Geometry: see drawing. Coordinates: mm, zero at the bounding-box minimum. A direction names the side the tool comes from. Coordinates: 2 decimals unless noted, no trailing zeros. Loops run counter-clockwise (first coordinate to the right, second up) from the corner with the lowest first, then second, coordinate; pieces in that order, holes last. Notation, with made-up numbers: (22.25, -1.5) -> (36.25, -1.5) arc R32 ccw to (36.25, 34.5) -> close; hole circle Ø9 at (43.25, 31). An arc over 180 degrees is marked (long way). Put each result on its own line as item: value. Start each with the question number.
1) Cut plane C-C (y = 6). Return the cut outline in (x, z).
2) Material intervals for L1, parallel to X at y = 13, z = 2.5; L2, parallel to Y at x = 13, z = 3; L3, parallel to Y at x = 12.25, z = 2.2, sorted ascending.
3) Cut plane A-A (x = 12.5). Return the cut outline in (y, z), plus the area to 3 significant figures.
4) Cut plane D-D (x = 14.25). Return the cut outline in (y, z).
5) Cut plane B-B (z = 1.1). Return the cut outline in (x, y).
6) Contact query for flat-ended pins moving along their axis: P1, Ø1.6, axis at x = 14, z = 3, coming from the -Y side; P2, Ø2, axis at y = 7.5, z = 1.5, coming from the +X side; P3, Ø0.9, axis at y = 3.5, z = 2, coming from the -X side. Output: stop coordinate, or through.
7) Pull-direction query (Y, two-part tool) for the marked faces 1, 2, 3 and 4; classes: pulls with the +Y half, pulls with the -Y half, needs draft (parallel to the pull), parting line crosses it, or undercut.
8) Set-up query: the marked faces 5, 6 and 7. Return all of +Z, -Z, +X, -X, +Y, -Y with unobstructed straight access to the full face (end or side cutting, diameter ignored); none if empty.
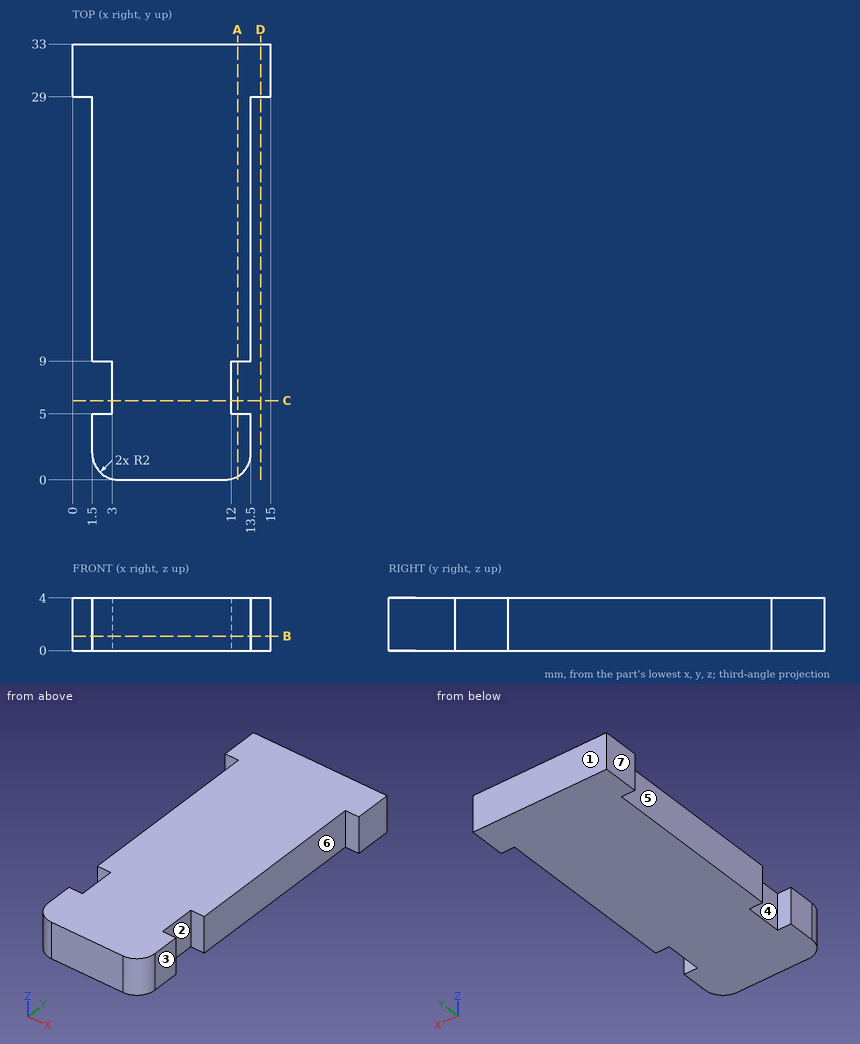
Results found:
1. outline: (3, 0) -> (12, 0) -> (12, 4) -> (3, 4) -> close
2. L1: x = 1.5 to 13.5
2. L2: y = 0.68 to 5, 9 to 33
2. L3: y = 0.15 to 5, 9 to 33
3. outline: (0.27, 0) -> (5, 0) -> (5, 4) -> (0.27, 4) -> close; (9, 0) -> (33, 0) -> (33, 4) -> (9, 4) -> close
3. area: 115 mm2
4. outline: (29, 0) -> (33, 0) -> (33, 4) -> (29, 4) -> close
5. outline: (0, 29) -> (1.5, 29) -> (1.5, 9) -> (3, 9) -> (3, 5) -> (1.5, 5) -> (1.5, 2) arc R2 ccw to (3.5, 0) -> (11.5, 0) arc R2 ccw to (13.5, 2) -> (13.5, 5) -> (12, 5) -> (12, 9) -> (13.5, 9) -> (13.5, 29) -> (15, 29) -> (15, 33) -> (0, 33) -> close
6. P1: stops at y = 0.95
6. P2: stops at x = 12
6. P3: stops at x = 1.5
7. face 1: pulls with the +Y half
7. face 2: undercut
7. face 3: needs draft
7. face 4: undercut
8. face 5: +Z, -Z, -X, -Y
8. face 6: +Z, -Z, +X, -Y
8. face 7: +Z, -Z, -X, +Y, -Y
